Read the model definition and answer for the solid it produces. Units are mm, in the model's axes. A direction names the side the tool comes from. Round coordinates to 2 decimals unless told otherwise and drop trailing zeros. Order: outer loops, then holes, each group sorted by start corner. A loop starts at its lowest first (then second) coordinate and runs counter-clockwise, first axis right, second up.
from build123d import *

# Parameters (mm, degrees)
PAD001_DEPTH         = 20.5
POCKET_DEPTH         = 17.8
SKETCH020_W          = 89.65
SKETCH020_H          = 5
POCKET002_DEPTH      = 12.8
HOLE006_D            = 5.3
HOLE006_CBORE_D      = 8.9
HOLE006_CBORE_DEPTH  = 5.4
SKETCH032_W          = 35
SKETCH032_H          = 37
POCKET010_DEPTH      = 101.001
SKETCH033_W          = 5
SKETCH033_H          = 15
POCKET011_DEPTH      = 20.501
POCKET011_DEPTH_BACK = 20.501
SKETCH034_R          = 1.2
POCKET012_DEPTH      = 103.501


with BuildPart() as part:
    # Sketch018 → Pad001 (new body, symmetric)
    with BuildSketch(Plane.XZ):
        Polygon((71.9, 102.9), (-23.5, 7.5), (-23.5, 0), (71.9, 0), (71.9, -10), (79.9, -10), (79.9, 102.9), align=None)
    extrude(amount=PAD001_DEPTH, both=True)

    # Sketch019 → Pocket (cut, symmetric)
    with BuildSketch(Plane.XZ):
        Polygon((-17.5, 4.5), (71.9, 4.5), (71.9, 104.5), (-27.5, 104.5), (-27.5, 14.5), align=None)
    extrude(amount=POCKET_DEPTH, both=True, mode=Mode.SUBTRACT)

    # Sketch020 → Pocket002 (cut, symmetric)
    with BuildSketch(Plane.XZ):
        with Locations((27.075, 2.5)):
            Rectangle(SKETCH020_W, SKETCH020_H)
    extrude(amount=POCKET002_DEPTH, both=True, mode=Mode.SUBTRACT)

    # Hole006 (through all)
    with Locations(Plane(origin=(71.9, 0, 0), x_dir=(0, 1, 0), z_dir=(-1, 0, 0))):
        with Locations((-12.5, -97), (12.5, -97), (-12.5, 5), (12.5, 5)):
            CounterBoreHole(HOLE006_D / 2, HOLE006_CBORE_D / 2, HOLE006_CBORE_DEPTH)

    # Sketch032 → Pocket010 (cut, through all)
    with BuildSketch(Plane.YZ.offset(77.5)):
        with Locations((0, 39.3)):
            Rectangle(SKETCH032_W, SKETCH032_H)
    extrude(amount=-POCKET010_DEPTH, mode=Mode.SUBTRACT)

    # Sketch033 → Pocket011 (cut, two sides)
    with BuildSketch(Plane.XZ) as pocket011_sk:
        with Locations((74.4, 41.5)):
            Rectangle(SKETCH033_W, SKETCH033_H)
    extrude(amount=-POCKET011_DEPTH, mode=Mode.SUBTRACT)
    extrude(pocket011_sk.sketch, amount=POCKET011_DEPTH_BACK, mode=Mode.SUBTRACT)

    # Sketch034 → Pocket012 (cut, through all)
    with BuildSketch(Plane.YZ.offset(80)):
        with Locations((-12.75, 52.94381)):
            Circle(SKETCH034_R)
        with Locations((12.75, 52.94381)):
            Circle(SKETCH034_R)
        with Locations((12.75, 25.94381)):
            Circle(SKETCH034_R)
        with Locations((-12.75, 25.94381)):
            Circle(SKETCH034_R)
        with BuildLine():
            ThreePointArc((-12.22, 46.66), (-13.97, 48.41), (-15.72, 46.66))
            Line((-15.72, 46.66), (-15.72, 36.5))
            ThreePointArc((-15.72, 36.5), (-13.97, 34.75), (-12.22, 36.5))
            Line((-12.22, 46.66), (-12.22, 36.5))
        make_face()
        with BuildLine():
            ThreePointArc((15.72, 46.66), (13.97, 48.41), (12.22, 46.66))
            Line((12.22, 46.66), (12.22, 36.5))
            ThreePointArc((12.22, 36.5), (13.97, 34.75), (15.72, 36.5))
            Line((15.72, 46.66), (15.72, 36.5))
        make_face()
        with BuildLine():
            Line((-7.62, 46.66), (-7.62, 32.3))
            ThreePointArc((-7.62, 32.3), (-7.248026, 31.401974), (-6.35, 31.03))
            Line((-6.35, 31.03), (6.35, 31.03))
            ThreePointArc((6.35, 31.03), (7.248026, 31.401974), (7.62, 32.3))
            Line((7.62, 32.3), (7.62, 46.66))
            ThreePointArc((7.62, 46.66), (7.248026, 47.558026), (6.35, 47.93))
            Line((6.35, 47.93), (-6.35, 47.93))
            ThreePointArc((-6.35, 47.93), (-7.248026, 47.558026), (-7.62, 46.66))
        make_face()
    extrude(amount=-POCKET012_DEPTH, mode=Mode.SUBTRACT)


solid = part.part
Q1. Straight lines are drawn through the part: probe 1 along Y at (x, z) = (79.1, 97); probe 2 along Z at (x, y) = (75, 12); probe 3 along Y at (x, z) = (12, 33). For each, find the intervals that lie inside material, in ascending order.
Outcome:
probe 1: y = -20.5 to -15.15, -9.85 to 9.85, 15.15 to 20.5
probe 2: z = -10 to -9.42, -0.58 to 20.8, 57.8 to 92.58, 101.42 to 102.9
probe 3: y = -20.5 to -17.8, 17.8 to 20.5
Q2. Flat-ended cylindrical pins translate along their axes: pin 1 (6 mm diameter, centred on y = 12.5, z = -5, fed in from -X); pin 2 (3 mm diameter, centred on x = 62, y = 15, fed in from +Z); pin 3 (4 mm diameter, centred on x = 49, y = -16.5, fed in from +Z). Find the tip coordinate at first contact, or state that the pin passes through.
Outcome:
pin 1: stops at x = 77.3
pin 2: stops at z = 4.5
pin 3: stops at z = 81.52
Q3. A cutting plane is placed at C-C, the plane y = 0. Give the vertices of the cut face in (x, z), plus the area to 3 significant figures.
Outcome:
outline: (-23.5, 0) - (-17.75, 0) - (-17.75, 4.75) - (-22, 9) - (-23.5, 7.5) - close; (71.9, -10) - (79.9, -10) - (79.9, 31.03) - (77.5, 31.03) - (77.5, 20.8) - (71.9, 20.8) - close; (71.9, 57.8) - (77.5, 57.8) - (77.5, 47.93) - (79.9, 47.93) - (79.9, 102.9) - (71.9, 102.9) - close
area: 697 mm2
Q4. For faces 3 (the face through (77.5, -8, 40)), 4 (the face through (78.72, -14.01, 34.75)), 5 (the face through (76.9, 19, 41)), determine the directions among +Z, -Z, +X, -X, +Y, -Y from which every point of the face is accessible in a straight line to the end or side of a thin tool.
Outcome:
face 3: -X
face 4: +X, -X
face 5: +Y, -Y
Q5. A cutting plane is placed at D-D, the plane z = 10.5. Give the vertices of the cut face in (x, y).
Outcome:
outline: (-20.5, -20.5) - (79.9, -20.5) - (79.9, 20.5) - (-20.5, 20.5) - (-20.5, 17.8) - (71.9, 17.8) - (71.9, -17.8) - (-20.5, -17.8) - close
Q6. A cutting plane is placed at B-B, the plane z = 97. Give the vertices of the cut face in (x, y).
Outcome:
outline: (66, -20.5) - (79.9, -20.5) - (79.9, -15.15) - (77.3, -15.15) - (77.3, -16.95) - (71.9, -16.95) - (71.9, -17.8) - (66, -17.8) - close; (66, 17.8) - (71.9, 17.8) - (71.9, 16.95) - (77.3, 16.95) - (77.3, 15.15) - (79.9, 15.15) - (79.9, 20.5) - (66, 20.5) - close; (71.9, -8.05) - (77.3, -8.05) - (77.3, -9.85) - (79.9, -9.85) - (79.9, 9.85) - (77.3, 9.85) - (77.3, 8.05) - (71.9, 8.05) - close
Q7. For a pull along Z with two mould halves and no side action, classify faces 1 (the face through (79, -12.22, 42)), 2 (the face through (71.9, 0, 82)) as released by +Z, released by -Z, zero draft, split by the parting line, or undercut.
Outcome:
face 1: undercut
face 2: zero draft
Q8. A cutting plane is placed at A-A, the plane x = 21. Give the vertices of the cut face in (y, z), plus the area to 3 significant figures.
Outcome:
outline: (-20.5, 0) - (-12.8, 0) - (-12.8, 4.5) - (-17.8, 4.5) - (-17.8, 52) - (-20.5, 52) - close; (12.8, 0) - (20.5, 0) - (20.5, 52) - (17.8, 52) - (17.8, 4.5) - (12.8, 4.5) - close
area: 326 mm2
